Read the model definition and answer for the solid it produces. Units are mm, in the model's axes. Round coordinates to 2 decimals unless told otherwise and drop trailing zeros. Loops run counter-clockwise (first coordinate to the right, second up) from the corner with the lowest first, then second, coordinate; pieces in that order, holes last. Notation, with made-up numbers: M 87.5,86 L 103.5,86 A35 cw 103.5,124 Z; hole C 45,41.5 d7. An arc over 180 degrees is marked long. Write each question's results on one line, items separated by ' | '.
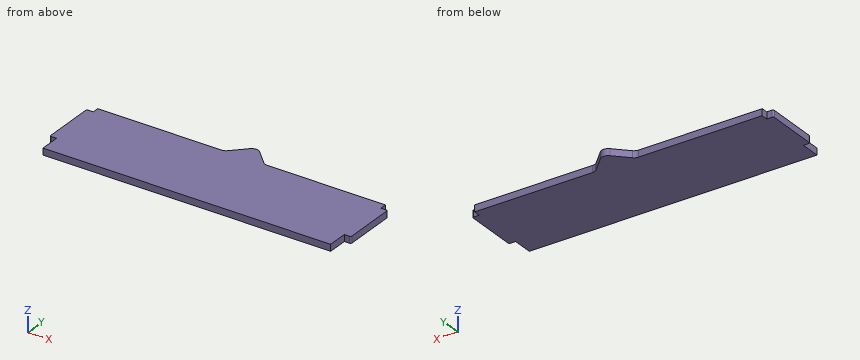
```python
from build123d import *

# Parameters (mm, degrees)
BOSS_EXTRUDE1_DEPTH = 5
FILLET1_R           = 5
FILLET2_R           = 1


with BuildPart() as part:
    # Sketch1 → Boss-Extrude1 (new body)
    with BuildSketch(Plane.XY):
        Polygon((215, 55.05), (215, 60), (124.595635172, 60), (109.595635172, 75), (94.595635172, 60), (0, 60), (0, 55.05), (-5, 55.05), (-5, 14.95), (0, 14.95), (0, 0), (215, 0), (215, 14.95), (220, 14.95), (220, 55.05), align=None)
    extrude(amount=BOSS_EXTRUDE1_DEPTH)

    # Fillet1
    fillet1_edges = [part.edges().sort_by_distance(p)[0] for p in [
        (94.595635172, 60, 2.5),
        (109.595635172, 75, 2.5),
        (124.595635172, 60, 2.5),
    ]]
    fillet(fillet1_edges, radius=FILLET1_R)

    # Fillet2
    fillet2_edges = [part.edges().sort_by_distance(p)[0] for p in [
        (-5, 14.95, 2.5),
        (-5, 55.05, 2.5),
        (220, 55.05, 2.5),
        (220, 14.95, 2.5),
    ]]
    fillet(fillet2_edges, radius=FILLET2_R)


solid = part.part
```
1. Find section C-C, the plane x = 145. Give the vertices of the cut face in (y, z), then the cut area to 3 significant figures.
Completed:
outline: M 0,0 L 60,0 L 60,5 L 0,5 Z | area: 300 mm2
2. Find the intervals of material crossed by L1, parallel to Y at x = 201.5, z = 1.85; L2, parallel to X at y = 57, z = 1.5; L3, parallel to X at y = 68, z = 1.6, in increasing order.
Completed:
L1: y = 0 to 60 | L2: x = 0 to 215 | L3: x = 102.6 to 116.6
3. Find section A-A, the plane z = 2.75. Give the vertices of the cut face in (x, y), then the cut area to 3 significant figures.
Completed:
outline: M -5,15.95 A1 ccw -4,14.95 L 0,14.95 L 0,0 L 215,0 L 215,14.95 L 219,14.95 A1 ccw 220,15.95 L 220,54.05 A1 ccw 219,55.05 L 215,55.05 L 215,60 L 126.67,60 A5 cw 123.13,61.46 L 113.13,71.46 A5 ccw 106.06,71.46 L 96.06,61.46 A5 cw 92.52,60 L 0,60 L 0,55.05 L -4,55.05 A1 ccw -5,54.05 Z | area: 13,500 mm2
4. Given P1, Ø1.5, axis at y = 6, z = 3, coming from the -X side; P2, Ø1.2, axis at x = 217.5, z = 3.5, coming from the -Y side; P3, Ø3, axis at x = 216, z = 3.5, coming from the +Y side, each flat-ended and moving along its own axis, determine where each tip first touches the part or whether it passes through.
Completed:
P1: stops at x = 0 | P2: stops at y = 14.95 | P3: stops at y = 60
5. Find section B-B, the plane y = 10. Give the vertices of the cut face in (x, z).
Completed:
outline: M 0,0 L 215,0 L 215,5 L 0,5 Z
